Geometry check sheet. Reference: the model listing, model coordinates, mm. A direction names the side the tool comes from. Coordinates: 2 decimals unless noted, no trailing zeros. Loops run counter-clockwise (first coordinate to the right, second up) from the corner with the lowest first, then second, coordinate; pieces in that order, holes last.
from build123d import *

# Parameters (mm, degrees)
F0_W     = 75
F0_H     = 75
F1_DEPTH = 2.5
F3_DEPTH = 2.5


with BuildPart() as f1:
    # F0 (on Top) → F1 (new body)
    with BuildSketch(Plane.XY):
        Rectangle(F0_W, F0_H)
    extrude(amount=-F1_DEPTH)

    # F2 (on Top) → F3 (cut, through all)
    with BuildSketch(Plane.XY):
        Polygon((-32.5, 13.75), (-32.5, 23.75), (-37.5, 21.25), (-37.5, 16.25), align=None)
        Polygon((-32.5, -13.75), (-37.5, -16.25), (-37.5, -21.25), (-32.5, -23.75), align=None)
        Polygon((37.5, 21.25), (32.5, 23.75), (32.5, 13.75), (37.5, 16.25), align=None)
        Polygon((32.5, -13.75), (32.5, -23.75), (37.5, -21.25), (37.5, -16.25), align=None)
        Polygon((-16.25, 37.5), (-21.25, 37.5), (-23.75, 32.5), (-13.75, 32.5), align=None)
        Polygon((21.25, 37.5), (16.25, 37.5), (13.75, 32.5), (23.75, 32.5), align=None)
        Polygon((-13.75, -32.5), (-23.75, -32.5), (-21.25, -37.5), (-16.25, -37.5), align=None)
        Polygon((16.25, -37.5), (21.25, -37.5), (23.75, -32.5), (13.75, -32.5), align=None)
    extrude(amount=-F3_DEPTH, mode=Mode.SUBTRACT)


solid = f1.part
(1) Draft check along Y on faces 1 (the flat face through (-37.5, 0, -1)), 2 (the flat face through (0, -37.5, -1)), 3 (the flat face through (-35, -22.5, -1.2)). Enter one of: +Y half, -Y half, draft (parallel to the pull), parting line (faces both ways), or undercut.
Findings:
face 1: draft
face 2: -Y half
face 3: undercut
(2) Access from +Z, -Z, +X, -X, +Y, -Y to the whole of each face (thin tool, end or side, straight path). Record for faces 4 (the flat face through (-1, 1, 0)), 5 (the flat face through (35, 15, -1)).
Findings:
face 4: +Z, +X, -X, +Y, -Y
face 5: +Z, -Z
(3) Gauge pin test, flat ends, axial feed: pin 1 Ø1.2 at (x, z) = (20.5, -1) entering from +Y; pin 2 Ø1.2 at (x, z) = (-17.5, -1) entering from -Y; pin 3 Ø0.8 at (y, z) = (18, -0.5) entering from -X. Record the tip position at first contact, or that the pin passes through.
Findings:
pin 1: stops at y = 32.5
pin 2: stops at y = -32.5
pin 3: stops at x = -32.5
(4) Scan lines: L1, parallel to Y at x = -22.5, z = -0.25; L2, parallel to X at y = -33, z = -1.5; L3, parallel to X at y = 23.5, z = -1.05. Record each from-to range of solid material in increasing order.
Findings:
L1: y = -37.5 to -35, -32.5 to 32.5, 35 to 37.5
L2: x = -37.5 to -23.5, -14 to 14, 23.5 to 37.5
L3: x = -37.5 to -33, -32.5 to 32.5, 33 to 37.5
(5) Sectioned sample at A-A on x = 20. Record the cut outline in (y, z), and give its area (4 significant figures).
Findings:
outline: (-32.5, -2.5) - (32.5, -2.5) - (32.5, 0) - (-32.5, 0) - close
area: 162.5 mm2
